from build123d import *

# Parameters (mm, degrees)
SKETCH1_W              = 15.796409329
SKETCH1_H              = 13.049207706
BOSS_EXTRUDE2_DEPTH    = 10
BOSS_EXTRUDE2_2_DEPTH  = 10
BOSS_EXTRUDE2_3_DEPTH  = 10
BOSS_EXTRUDE2_4_DEPTH  = 10
BOSS_EXTRUDE2_5_DEPTH  = 10
BOSS_EXTRUDE2_6_DEPTH  = 10
BOSS_EXTRUDE2_7_DEPTH  = 10
BOSS_EXTRUDE2_8_DEPTH  = 10
BOSS_EXTRUDE2_9_DEPTH  = 10
BOSS_EXTRUDE2_10_DEPTH = 10
BOSS_EXTRUDE2_11_DEPTH = 10
BOSS_EXTRUDE2_12_DEPTH = 10
SKETCH2_W              = 115.149189571
SKETCH2_H              = 60.247442975
BOSS_EXTRUDE3_DEPTH    = 10


with BuildPart() as part:
    # Sketch1 → Boss-Extrude2 (new body)
    with BuildSketch(Plane.XY):
        with Locations((-24.600632245, -22.14931308)):
            Rectangle(SKETCH1_W, SKETCH1_H)
    extrude(amount=BOSS_EXTRUDE2_DEPTH)



with BuildPart() as body_2:
    # Sketch1 → Boss-Extrude2 2 (new body)
    with BuildSketch(Plane.XY):
        with Locations((-54.600632245, -22.14931308)):
            Rectangle(SKETCH1_W, SKETCH1_H)
    extrude(amount=BOSS_EXTRUDE2_2_DEPTH)


with BuildPart() as body_3:
    # Sketch1 → Boss-Extrude2 3 (new body)
    with BuildSketch(Plane.XY):
        with Locations((5.399367756, -22.14931308)):
            Rectangle(SKETCH1_W, SKETCH1_H)
    extrude(amount=BOSS_EXTRUDE2_3_DEPTH)


with BuildPart() as body_4:
    # Sketch1 → Boss-Extrude2 4 (new body)
    with BuildSketch(Plane.XY):
        with Locations((35.399367756, -22.14931308)):
            Rectangle(SKETCH1_W, SKETCH1_H)
    extrude(amount=BOSS_EXTRUDE2_4_DEPTH)


with BuildPart() as body_5:
    # Sketch1 → Boss-Extrude2 5 (new body)
    with BuildSketch(Plane.XY):
        with Locations((-24.600632245, -2.14931308)):
            Rectangle(SKETCH1_W, SKETCH1_H)
    extrude(amount=BOSS_EXTRUDE2_5_DEPTH)


with BuildPart() as body_6:
    # Sketch1 → Boss-Extrude2 6 (new body)
    with BuildSketch(Plane.XY):
        with Locations((5.399367756, -2.14931308)):
            Rectangle(SKETCH1_W, SKETCH1_H)
    extrude(amount=BOSS_EXTRUDE2_6_DEPTH)


with BuildPart() as body_7:
    # Sketch1 → Boss-Extrude2 7 (new body)
    with BuildSketch(Plane.XY):
        with Locations((35.399367756, -2.14931308)):
            Rectangle(SKETCH1_W, SKETCH1_H)
    extrude(amount=BOSS_EXTRUDE2_7_DEPTH)


with BuildPart() as body_8:
    # Sketch1 → Boss-Extrude2 8 (new body)
    with BuildSketch(Plane.XY):
        with Locations((-24.600632245, 17.85068692)):
            Rectangle(SKETCH1_W, SKETCH1_H)
    extrude(amount=BOSS_EXTRUDE2_8_DEPTH)


with BuildPart() as body_9:
    # Sketch1 → Boss-Extrude2 9 (new body)
    with BuildSketch(Plane.XY):
        with Locations((5.399367756, 17.85068692)):
            Rectangle(SKETCH1_W, SKETCH1_H)
    extrude(amount=BOSS_EXTRUDE2_9_DEPTH)


with BuildPart() as body_10:
    # Sketch1 → Boss-Extrude2 10 (new body)
    with BuildSketch(Plane.XY):
        with Locations((35.399367756, 17.85068692)):
            Rectangle(SKETCH1_W, SKETCH1_H)
    extrude(amount=BOSS_EXTRUDE2_10_DEPTH)


with BuildPart() as body_11:
    # Sketch1 → Boss-Extrude2 11 (new body)
    with BuildSketch(Plane.XY):
        with Locations((-54.600632245, -2.14931308)):
            Rectangle(SKETCH1_W, SKETCH1_H)
    extrude(amount=BOSS_EXTRUDE2_11_DEPTH)


with BuildPart() as body_12:
    # Sketch1 → Boss-Extrude2 12 (new body)
    with BuildSketch(Plane.XY):
        with Locations((-54.600632245, 17.85068692)):
            Rectangle(SKETCH1_W, SKETCH1_H)
    extrude(amount=BOSS_EXTRUDE2_12_DEPTH)


with BuildPart() as part_1:
    add(part.part)

    add(body_2.part)  # Boss-Extrude3 merges body 2

    add(body_3.part)  # Boss-Extrude3 merges body 3

    add(body_4.part)  # Boss-Extrude3 merges body 4

    add(body_5.part)  # Boss-Extrude3 merges body 5

    add(body_6.part)  # Boss-Extrude3 merges body 6

    add(body_7.part)  # Boss-Extrude3 merges body 7

    add(body_8.part)  # Boss-Extrude3 merges body 8

    add(body_9.part)  # Boss-Extrude3 merges body 9

    add(body_10.part)  # Boss-Extrude3 merges body 10

    add(body_11.part)  # Boss-Extrude3 merges body 11

    add(body_12.part)  # Boss-Extrude3 merges body 12
    # Sketch2 → Boss-Extrude3 (add)
    with BuildSketch(Plane.XY):
        with Locations((-10.250784507, -3.160661043)):
            Rectangle(SKETCH2_W, SKETCH2_H)
    extrude(amount=-BOSS_EXTRUDE3_DEPTH)


solid = part_1.part
Input: part model. Units: mm. Frame: model coordinates. A direction names the side the tool comes from. Give positions to 0.01 mm unless a question says otherwise; leave off trailing zeros. Order: outer loops, then holes, each group sorted by start corner. A loop starts at its lowest first (then second) coordinate and runs counter-clockwise, first axis right, second up. Notation, with made-up numbers: (17.5, 37.25) - (63.5, 37.25) arc R24 cw to (63.5, 57.25) - close; hole circle Ø1 at (18, -16). An arc over 180 degrees is marked (long way). Answer as a JSON object with one key per item and string values. Group by question number.
Q1. Cut plane D-D, the plane x = 22.5. Output: boundary loops of the cut face in (y, z).
Q2. Line query: probe 1 along Y at (x, z) = (34.5, 8.25); probe 2 along X at (y, z) = (-20, 1.25); probe 3 along Z at (x, y) = (25.5, -13.5). Output: solid intervals per line, ascending.
Q3. Cut plane C-C, the plane z = 7.25. Count the separate pieces of the cut face and the enclosed holes in it, then the cut area to 3 significant figures.
Q4. Cut plane A-A, the plane x = 10.5. Output: boundary loops of the cut face in (y, z), then the cut area to 3 significant figures.
Q5. First-contact query: pin 1 Ø5 at (y, z) = (-23, 3) entering from -X; pin 2 Ø11 at (x, z) = (33.5, 6.5) entering from +Y; pin 3 Ø5 at (y, z) = (16, 7) entering from +X. Flat tips, straight axial feed; report the tip coordinate or a pass-through.
Q6. Mould query, pull axis Y, two halves, no side actions, for faces 6 (the face through (-25, -15.625, 5)), 7 (the face through (-25, -2, 10)), 8 (the face through (-11, -33.284, -5)). Classes: pulls with the +Y half, pulls with the -Y half, needs draft (parallel to the pull), parting line crosses it, or undercut.
Q7. Cut plane B-B, the plane y = 22.5. Output: boundary loops of the cut face in (x, z), then the cut area to 3 significant figures.
Q8. Set-up query: faces 1 (the face through (-62.499, -22, 5)), 2 (the face through (-25, -28.674, 5)), 3 (the face through (35, 24.375, 5)), 4 (the face through (35, -8.674, 5)), 5 (the face through (-2.499, -2, 5)). Return all of +Z, -Z, +X, -X, +Y, -Y with unobstructed straight access to the full face (end or side cutting, diameter ignored); none if empty.
Results:
{
 "1": {"outline": "(-33.28, -10) - (26.96, -10) - (26.96, 0) - (-33.28, 0) - close"},
 "2": {"probe 1": "-28.67 to -15.62, -8.67 to 4.38, 11.33 to 24.38", "probe 2": "-62.5 to -46.7, -32.5 to -16.7, -2.5 to 13.3, 27.5 to 43.3", "probe 3": "-10 to 0"},
 "3": {"separate pieces": "12", "enclosed holes": "0", "area": "2,470 mm^2"},
 "4": {"outline": "(-33.28, -10) - (26.96, -10) - (26.96, 0) - (24.38, 0) - (24.38, 10) - (11.33, 10) - (11.33, 0) - (4.38, 0) - (4.38, 10) - (-8.67, 10) - (-8.67, 0) - (-15.62, 0) - (-15.62, 10) - (-28.67, 10) - (-28.67, 0) - (-33.28, 0) - close", "area": "994 mm^2"},
 "5": {"pin 1": "x = -62.5", "pin 2": "y = 24.38", "pin 3": "x = 43.3"},
 "6": {"face 6": "undercut", "face 7": "needs draft", "face 8": "pulls with the -Y half"},
 "7": {"outline": "(-67.83, -10) - (47.32, -10) - (47.32, 0) - (43.3, 0) - (43.3, 10) - (27.5, 10) - (27.5, 0) - (13.3, 0) - (13.3, 10) - (-2.5, 10) - (-2.5, 0) - (-16.7, 0) - (-16.7, 10) - (-32.5, 10) - (-32.5, 0) - (-46.7, 0) - (-46.7, 10) - (-62.5, 10) - (-62.5, 0) - (-67.83, 0) - close", "area": "1,780 mm^2"},
 "8": {"face 1": "+Z, -X, +Y, -Y", "face 2": "+Z, +X, -X, -Y", "face 3": "+Z, +X, -X, +Y", "face 4": "+Z, +X, -X", "face 5": "+Z, +Y, -Y"}
}
